Drawing for the job (mm, zero at the part's lowest x, y, z). Coordinates: 2 decimals unless noted, no trailing zeros. Write each loop counter-clockwise with the first axis right and the second up, starting at its lowest first coordinate (ties: lowest second). Pieces come first, ordered by that corner, then holes. Notation, with made-up numbers: (-31, 34) -> (-3, 34) arc R9 ccw to (-3, 48) -> close; hole circle Ø7 at (40, 14.5). An arc over 180 degrees is marked (long way). Answer as CSV lines item,"result". Start each with the question number.
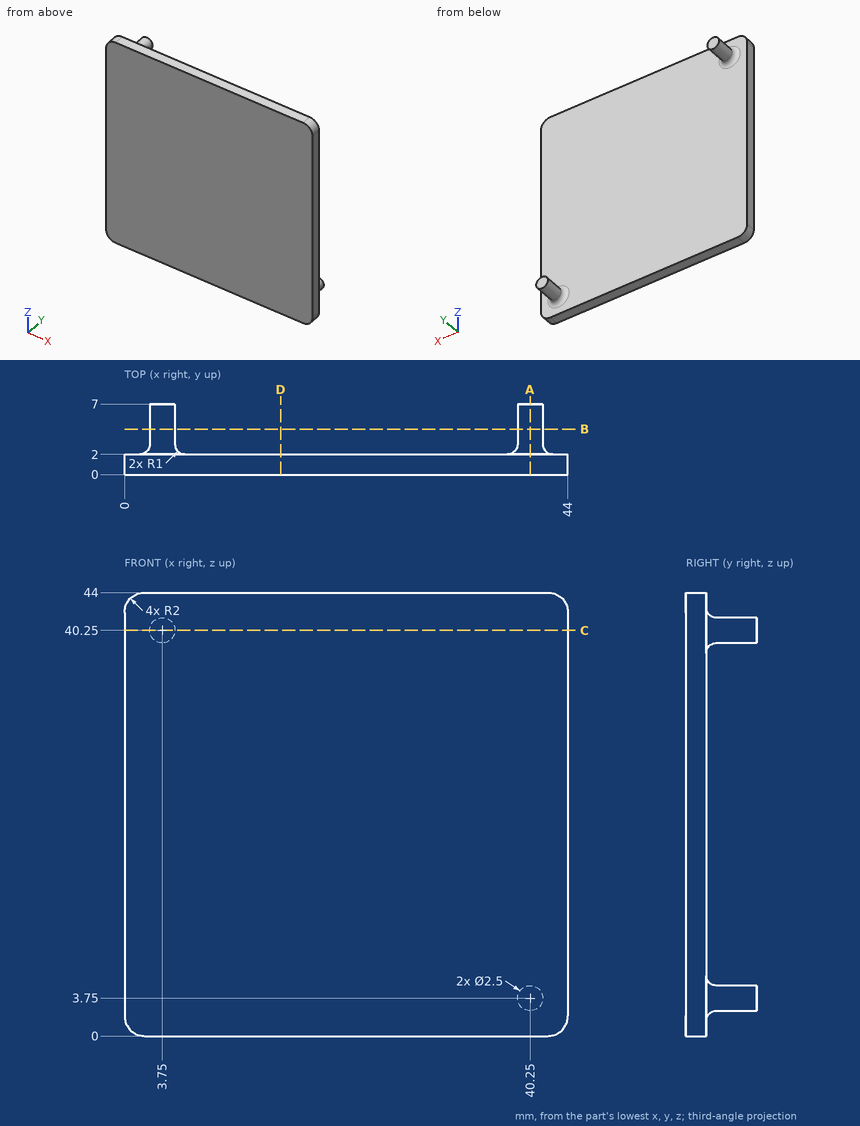
1. Cut at B-B (y = 4.5). Give the cut face in (x, z).
2. Wall check: line 1 (Y direction, x = 4, z = 37); line 2 (Y direction, x = 5.5, z = 40.5). Give the ranges that are in metal, low to high.
3. Cut at C-C (z = 40.25). Give the cut face in (x, y), then the cut area to 3 significant figures.
4. Cut at D-D (x = 15.5). Give the cut face in (y, z), then the cut area to 3 significant figures.
5. Flat gauge pins, fed straight in: P1, Ø10, axis at x = 26.5, z = 12, coming from the +Y side; P2, Ø4, axis at x = 12, z = 10, coming from the -Y side. Where does each tip first touch, or does it go through?
6. Cut at A-A (x = 40.25). Give the cut face in (y, z), then the cut area to 3 significant figures.
Geometry check:
1,outline,"circle Ø2.5 at (3.75, 40.25); circle Ø2.5 at (40.25, 3.75)"
2,line 1,"0 to 2"
2,line 2,"0 to 2.12"
3,outline,"(0, 0) -> (44, 0) -> (44, 2) -> (6, 2) arc R1 cw to (5, 3) -> (5, 7) -> (2.5, 7) -> (2.5, 3) arc R1 cw to (1.5, 2) -> (0, 2) -> close"
3,area,"101 mm²"
4,outline,"(0, 0) -> (2, 0) -> (2, 44) -> (0, 44) -> close"
4,area,"88.0 mm²"
5,P1,"y = 2"
5,P2,"y = 0"
6,outline,"(0, 0) -> (2, 0) -> (2, 1.5) arc R1 cw to (3, 2.5) -> (7, 2.5) -> (7, 5) -> (3, 5) arc R1 cw to (2, 6) -> (2, 44) -> (0, 44) -> close"
6,area,"101 mm²"
